Part print with two shaded views. Sizes in mm from the minimum x, y, z corner. Give positions to 0.01 mm unless a question says otherwise; leave off trailing zeros. Write each loop counter-clockwise with the first axis right and the second up, starting at its lowest first coordinate (ties: lowest second). Pieces come first, ordered by that corner, then holes.
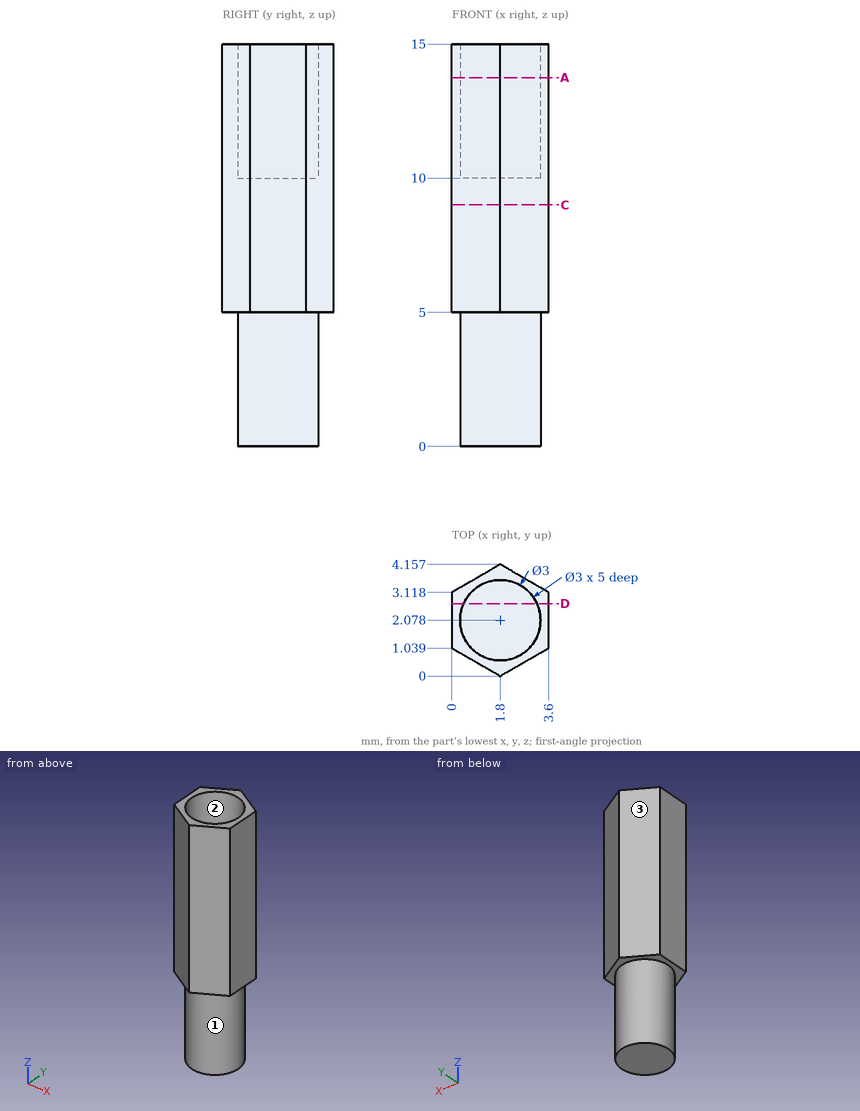
1) Flat gauge pins, fed straight in: P1, Ø1.8, axis at x = 2.5, y = 2.5, coming from the -Z side; P2, Ø1, axis at x = 0.5, z = 13, coming from the -Y side. Where does each tip first touch, or does it go through?
Check result:
P1: stops at z = 0
P2: stops at y = 0.46
2) Saw through at A-A (z = 13.75). Write the cut outline in (x, y).
Check result:
outline: (0, 1.04) - (1.8, 0) - (3.6, 1.04) - (3.6, 3.12) - (1.8, 4.16) - (0, 3.12) - close; hole circle Ø3 at (1.8, 2.08)
3) Saw through at C-C (z = 9). Write the cut outline in (x, y), and give its area (3 significant figures).
Check result:
outline: (0, 1.04) - (1.8, 0) - (3.6, 1.04) - (3.6, 3.12) - (1.8, 4.16) - (0, 3.12) - close
area: 11.2 mm2
4) Drill centre lines: L1, parallel to Z at x = 0.45, y = 1.95; L2, parallel to Z at x = 2, y = 3.8; L3, parallel to X at y = 2.3, z = 13.5. Where is each one in solid material? Low to high.
Check result:
L1: z = 0 to 10
L2: z = 5 to 15
L3: x = 0 to 0.32, 3.28 to 3.6
5) Mould opens along X. For the marked faces 1, 2 and 3 say: +X half, -X half, draft (parallel to the pull), parting line (faces both ways), or undercut.
Check result:
face 1: parting line
face 2: undercut
face 3: -X half
6) Saw through at D-D (y = 2.7). Write the cut outline in (x, z) (1 decimal), and give its area (3 significant figures).
Check result:
outline: (0, 5) - (0.4, 5) - (0.4, 0) - (3.2, 0) - (3.2, 5) - (3.6, 5) - (3.6, 15) - (3.2, 15) - (3.2, 10) - (0.4, 10) - (0.4, 15) - (0, 15) - close
area: 36.0 mm2
